Could you check a few things on this model? Use its own coordinates, in mm. A direction names the side the tool comes from. Coordinates: 2 decimals unless noted, no trailing zeros. Order: outer loops, then holes, each group sorted by start corner. A loop starts at its lowest first (then second) coordinate and runs counter-clockwise, first axis right, second up. Notation, with made-up numbers: (20, 89) - (42, 89) arc R31 ccw to (42, 114) - close; hole circle Ø7 at (7.5, 85.25). An arc over 180 degrees is marked (long way). One line per item, written item: value.
from build123d import *

# Parameters (mm, degrees)
ESQUISSE1_W             = 80
ESQUISSE1_H             = 80
BOSS_EXTRU_1_DEPTH      = 2
ESQUISSE2_R             = 24.5
BOSS_EXTRU_2_DEPTH      = 1
ESQUISSE3_R             = 2.05
ENL_V_MAT_EXTRU_1_DEPTH = 4
CHANFREIN1_SIZE         = 1.75
CHANFREIN1_SIZE2        = 2.594481695
ESQUISSE4_R             = 37.5
ESQUISSE4_R_2           = 35
BOSS_EXTRU_3_DEPTH      = 5
ESQUISSE5_W             = 80
ESQUISSE5_H             = 3
ENL_V_MAT_EXTRU_2_DEPTH = 8
ESQUISSE6_W             = 10
ESQUISSE6_H             = 10
ESQUISSE6_H_2           = 7
ENL_V_MAT_EXTRU_3_DEPTH = 8


with BuildPart() as part:
    # Esquisse1 → Boss.-Extru.1 (new body)
    with BuildSketch(Plane.XY):
        with Locations((40, 40)):
            Rectangle(ESQUISSE1_W, ESQUISSE1_H)
    extrude(amount=BOSS_EXTRU_1_DEPTH)

    # Esquisse2 → Boss.-Extru.2 (add)
    with BuildSketch(Plane.XY.offset(2)):
        with Locations((40, 40)):
            Circle(ESQUISSE2_R)
    extrude(amount=BOSS_EXTRU_2_DEPTH)

    # Esquisse3 → Enlèv. mat.-Extru.1 (cut, through all)
    with BuildSketch(Plane(origin=(0, 0, 0), x_dir=(-1, 0, 0), z_dir=(0, 0, -1))):
        with Locations((-50, 50)):
            Circle(ESQUISSE3_R)
        with Locations((-50, 30)):
            Circle(ESQUISSE3_R)
        with Locations((-30, 30)):
            Circle(ESQUISSE3_R)
        with Locations((-30, 50)):
            Circle(ESQUISSE3_R)
    extrude(amount=-ENL_V_MAT_EXTRU_1_DEPTH, mode=Mode.SUBTRACT)

    # Chanfrein1
    chanfrein1_edges = [part.edges().sort_by_distance(p)[0] for p in [
        (52.05, 50, 0),
        (52.05, 30, 0),
        (32.05, 30, 0),
        (32.05, 50, 0),
    ]]
    chanfrein1_side = [part.faces().sort_by_distance(p)[0] for p in [
        (40, 40, 0),
    ]]
    chamfer(chanfrein1_edges, length=CHANFREIN1_SIZE, length2=CHANFREIN1_SIZE2, reference=chanfrein1_side[0])

    # Esquisse4 → Boss.-Extru.3 (add)
    with BuildSketch(Plane.XY.offset(2)):
        with Locations((40, 40)):
            Circle(ESQUISSE4_R)
        with Locations((40, 40)):
            Circle(ESQUISSE4_R_2, mode=Mode.SUBTRACT)
    extrude(amount=BOSS_EXTRU_3_DEPTH)

    # Esquisse5 → Enlèv. mat.-Extru.2 (cut, through all)
    with BuildSketch(Plane(origin=(0, 0, 0), x_dir=(-1, 0, 0), z_dir=(0, 0, -1))):
        with Locations((-40, 1.5)):
            Rectangle(ESQUISSE5_W, ESQUISSE5_H)
    extrude(amount=-ENL_V_MAT_EXTRU_2_DEPTH, mode=Mode.SUBTRACT)

    # Esquisse6 → Enlèv. mat.-Extru.3 (cut, through all)
    with BuildSketch(Plane(origin=(0, 0, 0), x_dir=(-1, 0, 0), z_dir=(0, 0, -1))):
        with Locations((-75, 75)):
            Rectangle(ESQUISSE6_W, ESQUISSE6_H)
        with Locations((-5, 75)):
            Rectangle(ESQUISSE6_W, ESQUISSE6_H)
        with Locations((-5, 6.5)):
            Rectangle(ESQUISSE6_W, ESQUISSE6_H_2)
        with Locations((-75, 6.5)):
            Rectangle(ESQUISSE6_W, ESQUISSE6_H_2)
    extrude(amount=-ENL_V_MAT_EXTRU_3_DEPTH, mode=Mode.SUBTRACT)


solid = part.part
Item 1: I want a section at D-D on x = 40. Please give me the cut outline in (y, z), then the cut area to 4 significant figures.
Conclusion:
outline: (3, 0) - (80, 0) - (80, 2) - (77.5, 2) - (77.5, 7) - (75, 7) - (75, 2) - (64.5, 2) - (64.5, 3) - (15.5, 3) - (15.5, 2) - (5, 2) - (5, 7) - (3, 7) - close
area: 225.5 mm²
Item 2: I'm going to push flat-ended pins straight in: pin 1 Ø1 at (x, y) = (33, 65.5) entering from +Z; pin 2 Ø1 at (y, z) = (76, 1) entering from +X; pin 3 Ø2 at (x, z) = (75, 0.5) entering from -Y. Where does each tip first touch, or does it pass through?
Conclusion:
pin 1: z = 2
pin 2: x = 70
pin 3: y = 10
Item 3: I want a section at B-B on x = 30. Please give me the cut outline in (y, z), then the cut area to 3 significant figures.
Conclusion:
outline: (3, 0) - (26.2, 0) - (27.95, 2.59) - (27.95, 3) - (17.63, 3) - (17.63, 2) - (6.46, 2) - (6.46, 7) - (3.86, 7) - (3.86, 2) - (3, 2) - close; (32.05, 2.59) - (33.8, 0) - (46.2, 0) - (47.95, 2.59) - (47.95, 3) - (32.05, 3) - close; (52.05, 2.59) - (53.8, 0) - (80, 0) - (80, 2) - (76.14, 2) - (76.14, 7) - (73.54, 7) - (73.54, 2) - (62.37, 2) - (62.37, 3) - (52.05, 3) - close
area: 191 mm²
Item 4: For faces 5 (the face through (51.5, 31.4, 2.8)), 6 (the face through (5, 10, 1)), 7 (the face through (41.563, 77.467, 4.465)), 8 (the face through (0, 40, 1)), 9 (the face through (70, 75, 1)), which set-ups out of +Z, -Z, +X, -X, +Y, -Y let a thin tool reach every point of the face, with its end or its side?
Conclusion:
face 5: +Z, -Z
face 6: +Z, -Z, -X, -Y
face 7: +Z
face 8: +Z, -Z, -X, +Y, -Y
face 9: +Z, -Z, +X, +Y
Item 5: Thinking about a two-plate mould opening in X: for faces 1 (the face through (70, 6, 1)), 2 (the face through (40, 3, 2)), 3 (the face through (30.267, 32.033, 2.794)), 4 (the face through (40, 40, 3)), which applies, pulls with the +X half, pulls with the -X half, needs draft (parallel to the pull), parting line crosses it, or undercut?
Conclusion:
face 1: pulls with the +X half
face 2: needs draft
face 3: undercut
face 4: undercut
Item 6: I want a section at A-A on y = 40. Please give me the cut outline in (x, z).
Conclusion:
outline: (0, 0) - (80, 0) - (80, 2) - (77.5, 2) - (77.5, 7) - (75, 7) - (75, 2) - (64.5, 2) - (64.5, 3) - (15.5, 3) - (15.5, 2) - (5, 2) - (5, 7) - (2.5, 7) - (2.5, 2) - (0, 2) - close
Item 7: I want a section at C-C on y = 50. Please give me the cut outline in (x, z).
Conclusion:
outline: (0, 0) - (26.2, 0) - (27.95, 2.59) - (27.95, 3) - (17.63, 3) - (17.63, 2) - (6.46, 2) - (6.46, 7) - (3.86, 7) - (3.86, 2) - (0, 2) - close; (32.05, 2.59) - (33.8, 0) - (46.2, 0) - (47.95, 2.59) - (47.95, 3) - (32.05, 3) - close; (52.05, 2.59) - (53.8, 0) - (80, 0) - (80, 2) - (76.14, 2) - (76.14, 7) - (73.54, 7) - (73.54, 2) - (62.37, 2) - (62.37, 3) - (52.05, 3) - close
Item 8: If I drill on probe 1 along Y at (x, z) = (50, 2.9); probe 2 along Y at (x, z) = (40, 5.75); probe 3 along Z at (x, y) = (43, 6), over which ranges is the centre line in solid material (lowest first)?
Conclusion:
probe 1: 3.86 to 6.46, 17.63 to 27.95, 32.05 to 47.95, 52.05 to 62.37, 73.54 to 76.14
probe 2: 3 to 5, 75 to 77.5
probe 3: 0 to 2
